```python
from build123d import *

# Parameters (mm, degrees)
SKETCH2_R              = 10
CUT_EXTRUDE1_DEPTH     = 76
M24_TAPPED_HOLE3_D     = 21
M24_TAPPED_HOLE3_DEPTH = 27
M24_TAPPED_HOLE3_TIP   = 6.3090365
M12_TAPPED_HOLE1_D     = 10.2
M12_TAPPED_HOLE1_DEPTH = 15
M12_TAPPED_HOLE1_TIP   = 3.064389157


with BuildPart() as part:
    # Sketch1 → Revolve1 (revolve)
    with BuildSketch(Plane(origin=(0, 0, 0), x_dir=(0, 0, -1), z_dir=(1, 0, 0))):
        with BuildLine():
            Line((14, 0), (35, 0))
            Line((35, 0), (81, 47))
            Line((81, 47), (81, 53))
            Line((81, 53), (138, 53))
            Line((138, 53), (138, 75))
            Line((138, 75), (94, 75))
            ThreePointArc((94, 75), (89.757359313, 76.757359313), (88, 81))
            Line((88, 81), (28, 81))
            Line((28, 81), (28, 33))
            Line((28, 33), (14, 24.917096231))
            Line((14, 24.917096231), (14, 0))
        make_face()
    revolve(axis=Axis((0, 40.822828071, 0), (0, -1, 0)))

    # Sketch2 → Cut-Extrude1 (cut, through all)
    with BuildSketch(Plane(origin=(0, 75, 0), x_dir=(1, 0, 0), z_dir=(0, 1, 0))):
        with Locations((0, 112.5)):
            Circle(SKETCH2_R)
        with Locations((97.427857926, 56.25)):
            Circle(SKETCH2_R)
        with Locations((97.427857926, -56.25)):
            Circle(SKETCH2_R)
        with Locations((0, -112.5)):
            Circle(SKETCH2_R)
        with Locations((-97.427857926, -56.25)):
            Circle(SKETCH2_R)
        with Locations((-97.427857926, 56.25)):
            Circle(SKETCH2_R)
    extrude(amount=-CUT_EXTRUDE1_DEPTH, mode=Mode.SUBTRACT)

    # M24 Tapped Hole3
    with Locations(Plane(origin=(0, 81, 0), x_dir=(1, 0, 0), z_dir=(0, 1, 0))):
        with Locations((0, 60), (0, -60), (-5.787213998, -5.032102647)):
            Hole(M24_TAPPED_HOLE3_D / 2, depth=M24_TAPPED_HOLE3_DEPTH)
            with Locations((0, 0, -(M24_TAPPED_HOLE3_DEPTH + M24_TAPPED_HOLE3_TIP / 2))):  # 118° drill point
                Cone(0, M24_TAPPED_HOLE3_D / 2, M24_TAPPED_HOLE3_TIP, mode=Mode.SUBTRACT)

    # M12 Tapped Hole1
    with Locations(Plane(origin=(0, 81, 0), x_dir=(1, 0, 0), z_dir=(0, 1, 0))):
        with Locations((-44, 0), (44, 0)):
            Hole(M12_TAPPED_HOLE1_D / 2, depth=M12_TAPPED_HOLE1_DEPTH)
            with Locations((0, 0, -(M12_TAPPED_HOLE1_DEPTH + M12_TAPPED_HOLE1_TIP / 2))):  # 118° drill point
                Cone(0, M12_TAPPED_HOLE1_D / 2, M12_TAPPED_HOLE1_TIP, mode=Mode.SUBTRACT)


solid = part.part
```
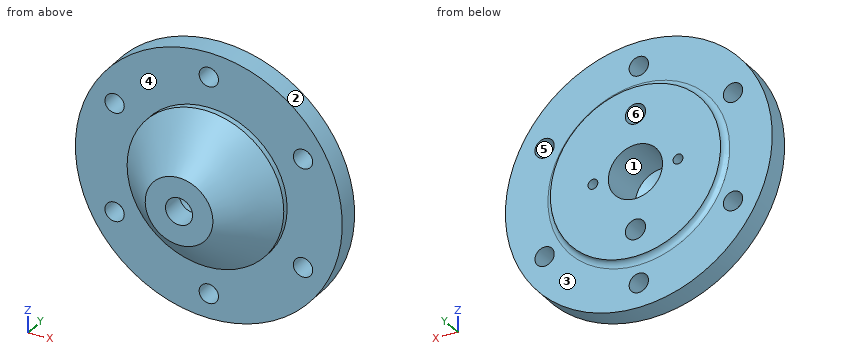
Geometry check sheet. Reference: the model listing, model coordinates, mm. Face numbers are marked on the shaded views. A direction names the side the tool comes from. Coordinates: 2 decimals unless noted, no trailing zeros. Order: outer loops, then holes, each group sorted by start corner. A loop starts at its lowest first (then second) coordinate and runs counter-clockwise, first axis right, second up.
Item 1: Section check B-B (y = 10). Enter the section's corners in (x, z), plus the area to 3 significant figures.
Item 2: Section check C-C (z = 56.25). Count the separate pieces of the cut face and the enclosed holes in it, plus the area to 3 significant figures.
Item 3: Section check A-A (z = -112.5). Enter the section's corners in (x, y), plus the area to 3 significant figures.
Item 4: Tool access check on the marked faces 4, 5 and 6. Record the directions out of +Z, -Z, +X, -X, +Y, -Y that give a thin tool (end or side, any length) a straight path to the whole face; none if there is none.
Item 5: Scan lines: line 1 along X through (y, z) = (61, -64); line 2 along Z through (x, y) = (-95.5, 58); line 3 along Y through (x, z) = (65, -70). Record each from-to range of solid material in increasing order.
Item 6: Depth check by flat-ended pin: pin 1 (1.5 mm diameter, centred on x = 0.5, z = 49.5, fed in from -Y); pin 2 (1 mm diameter, centred on y = 42, z = -35.5, fed in from +X); pin 3 (8 mm diameter, centred on x = 43, y = 43, fed in from +Z); pin 4 (13.5 mm diameter, centred on x = 44, z = 0, fed in from +Y). Enter the tip coordinate at first touch or a pass-through.
Item 7: Mould release check, pull along X, two halves, no side actions. Record for the marked faces 1, 2 and 3: released by +X, released by -X, zero draft, split by the parting line, or undercut.
Check sheet entries:
1. outline: circle Ø89.57 at (0, 0); hole circle Ø28 at (0, 0)
1. area: 5,690 mm2
2. separate pieces: 3
2. enclosed holes: 0
2. area: 7,510 mm2
3. outline: (-79.92, 53) - (-10, 53) - (-10, 75) - (-79.92, 75) - close; (10, 53) - (79.92, 53) - (79.92, 75) - (10, 75) - close
3. area: 3,080 mm2
4. face 4: -Y
4. face 5: +Y, -Y
4. face 6: +Y
5. line 1: x = -122.26 to -103.75, -91.11 to -9.71, 9.71 to 91.11, 103.75 to 122.26
5. line 2: z = -99.62 to -66.06, -46.44 to 46.44, 66.06 to 99.62
5. line 3: y = 53 to 75
6. pin 1: stops at y = 14.05
6. pin 2: stops at x = 67.93
6. pin 3: stops at z = 69.25
6. pin 4: stops at y = 81
7. face 1: undercut
7. face 2: split by the parting line
7. face 3: zero draft
